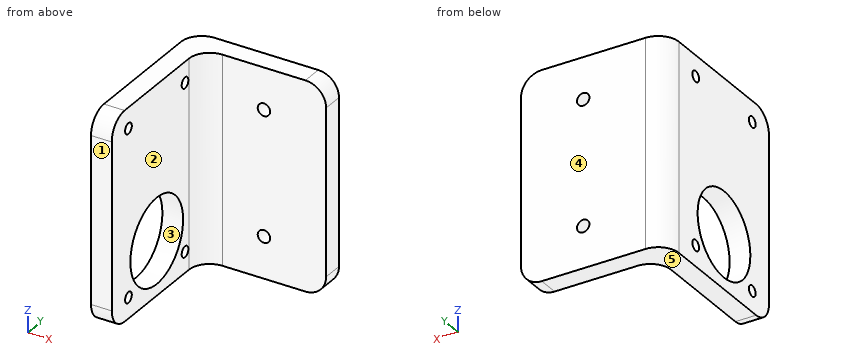
```python
from build123d import *

# Parameters (mm, degrees)
ESQUISSE1_W             = 30
ESQUISSE1_H             = 50
BOSS_EXTRU_1_DEPTH      = 5
ESQUISSE2_W             = 50
ESQUISSE2_H             = 40
BOSS_EXTRU_2_DEPTH      = 5
CONG_2_R                = 5
ESQUISSE11_R            = 1.5
ENL_V_MAT_EXTRU_2_DEPTH = 52.23475383
ESQUISSE12_R            = 10.25
ESQUISSE12_R_2          = 1.3
ENL_V_MAT_EXTRU_3_DEPTH = 59.736700622


with BuildPart() as part:
    # Esquisse1 → Boss.-Extru.1 (new body)
    with BuildSketch(Plane(origin=(0, 0, 0), x_dir=(1, 0, 0), z_dir=(0, 1, 0))):
        Rectangle(ESQUISSE1_W, ESQUISSE1_H)
    extrude(amount=-BOSS_EXTRU_1_DEPTH)

    # Esquisse2 → Boss.-Extru.2 (add)
    with BuildSketch(Plane.ZY.offset(15)):
        with Locations((0, -20)):
            Rectangle(ESQUISSE2_W, ESQUISSE2_H)
    extrude(amount=BOSS_EXTRU_2_DEPTH)

    # Congé2
    cong_2_edges = [part.edges().sort_by_distance(p)[0] for p in [
        (-15, -5, 0),
        (-17.5, -40, 25),
        (-17.5, -40, -25),
        (-20, 0, 0),
        (15, -2.5, 25),
        (15, -2.5, -25),
    ]]
    fillet(cong_2_edges, radius=CONG_2_R)

    # Esquisse11 → Enlèv. mat.-Extru.2 (cut, through all)
    with BuildSketch(Plane(origin=(0, 0, 0), x_dir=(1, 0, 0), z_dir=(0, 1, 0))):
        with Locations(Location((0, 15, 0), (0, 0, 270))):
            Circle(ESQUISSE11_R)
        with Locations(Location((0, -15, 0), (0, 0, 270))):
            Circle(ESQUISSE11_R)
    extrude(amount=-ENL_V_MAT_EXTRU_2_DEPTH, mode=Mode.SUBTRACT)

    # Esquisse12 → Enlèv. mat.-Extru.3 (cut, through all)
    with BuildSketch(Plane.ZY.offset(20)):
        with Locations((-12, -22.5)):
            Circle(ESQUISSE12_R)
        with Locations((-20, -11.5)):
            Circle(ESQUISSE12_R_2)
        with Locations((-20, -33.5)):
            Circle(ESQUISSE12_R_2)
        with Locations((20, -33.5)):
            Circle(ESQUISSE12_R_2)
        with Locations((20, -11.5)):
            Circle(ESQUISSE12_R_2)
    extrude(amount=-ENL_V_MAT_EXTRU_3_DEPTH, mode=Mode.SUBTRACT)


solid = part.part
```
The model under review builds one solid part; all positions refer to its coordinate system, in mm. Face numbers are marked on the shaded views. A direction names the side the tool comes from. Round coordinates to 2 decimals unless told otherwise and drop trailing zeros. Order: outer loops, then holes, each group sorted by start corner. A loop starts at its lowest first (then second) coordinate and runs counter-clockwise, first axis right, second up. Notation, with made-up numbers: (60.25, 43.25) - (65.25, 43.25) arc R24 cw to (65.25, 54.25) - close; hole circle Ø4 at (72, 82.5). An arc over 180 degrees is marked (long way). Answer in a Markdown table with one row per item.
(1) Clearance check with flat-ended pins moving along their axes: P1, Ø1.5, axis at y = -31.5, z = 0, coming from the +X side; P2, Ø4, axis at x = 0, z = 15, coming from the -Y side. State where each tip first meets the part, or that it passes through.
Result set:
| item | result |
|---|---|
| P1 | stops at x = -15 |
| P2 | stops at y = -5 |
(2) Mouldability with a two-part tool opening along Y and no side actions: class the marked faces 3, 4 and 5 as released by +Y, released by -Y, zero draft, split by the parting line, or undercut.
Result set:
| item | result |
|---|---|
| face 3 | undercut |
| face 4 | released by +Y |
| face 5 | zero draft |
(3) Take a section at C-C on y = -22.5. Write out the cut boundary in (x, z), plus the area to 4 significant figures.
Result set:
| item | result |
|---|---|
| outline | (-20, -25) - (-15, -25) - (-15, -22.25) - (-20, -22.25) - close; (-20, -1.75) - (-15, -1.75) - (-15, 25) - (-20, 25) - close |
| area | 147.5 mm2 |
(4) Take a section at B-B on z = 15. Write out the cut boundary in (x, y).
Result set:
| item | result |
|---|---|
| outline | (-20, -40) - (-15, -40) - (-15, -10) arc R5 cw to (-10, -5) - (-1.5, -5) - (-1.5, 0) - (-15, 0) arc R5 ccw to (-20, -5) - close; (1.5, -5) - (15, -5) - (15, 0) - (1.5, 0) - close |
(5) Machinability: for the marked faces 1 and 2, which of the approach directions +Z, -Z, +X, -X, +Y, -Y give a long, thin tool a straight path to every point of the face, cutting with its end or side? Answer none if there is none.
Result set:
| item | result |
|---|---|
| face 1 | +Z, -Z, +X, -X, -Y |
| face 2 | +Z, -Z, +X, -Y |
(6) Take a section at A-A on y = -11.5. Write out the cut boundary in (x, z), plus the area to 3 significant figures.
Result set:
| item | result |
|---|---|
| outline | (-20, -25) - (-15, -25) - (-15, -21.3) - (-20, -21.3) - close; (-20, -18.7) - (-15, -18.7) - (-15, 18.7) - (-20, 18.7) - close; (-20, 21.3) - (-15, 21.3) - (-15, 25) - (-20, 25) - close |
| area | 224 mm2 |
(7) For line 1 (Z direction, x = -17, y = -22); line 2 (Y direction, x = -17, z = -20); line 3 (X direction, y = -37, z = 12), list the stretches that pass through material, from the lowest coordinate up. Write a range as from..to.
Result set:
| item | result |
|---|---|
| line 1 | z = -25..-22.24, -1.76..25 |
| line 2 | y = -40..-34.8, -32.2..-28.91, -16.09..-12.8, -10.2..-0.42 |
| line 3 | x = -20..-15 |
(8) Take a section at D-D on z = 4. Write out the cut boundary in (x, y), plus the area to 3 significant figures.
Result set:
| item | result |
|---|---|
| outline | (-20, -40) - (-15, -40) - (-15, -10) arc R5 cw to (-10, -5) - (15, -5) - (15, 0) - (-15, 0) arc R5 ccw to (-20, -5) - close |
| area | 350 mm2 |
